Verification items for the finished model (mm, model axes). A direction names the side the tool comes from. Round coordinates to 2 decimals unless told otherwise and drop trailing zeros. Order: outer loops, then holes, each group sorted by start corner. A loop starts at its lowest first (then second) coordinate and runs counter-clockwise, first axis right, second up. Notation, with made-up numbers: (7.25, 74) -> (66.25, 74) arc R25 cw to (66.25, 97) -> close; hole circle Ø11 at (22.5, -11). An arc over 180 degrees is marked (long way). Answer in a Markdown table with one row per item. Add a question column.
```python
from build123d import *

# Parameters (mm, degrees)
EXTRUDE_1_DEPTH     = 15
CUT_EXTRUDE_1_DEPTH = 14
SKETCH_7_W          = 48
SKETCH_7_H          = 6
CUT_EXTRUDE_2_DEPTH = 1
SKETCH_8_W          = 14
SKETCH_8_H          = 4
CUT_EXTRUDE_3_DEPTH = 1


with BuildPart() as part:
    # 草图3 → 凸台-拉伸1 (new body)
    with BuildSketch(Plane.XY):
        Polygon((-26, 21.5), (24, 21.5), (24, 13.5), (6.5, 13.5), (6.5, 8), (17.5, 8), (17.5, -1), (12.5, -1), (12.5, -17.5), (-12.5, -17.5), (-12.5, -1), (-17.5, -1), (-17.5, 8), (-11.75, 8), (-11.75, 13.5), (-26, 13.5), align=None)
    extrude(amount=EXTRUDE_1_DEPTH)

    # 草图4 → 切除-拉伸1 (cut)
    with BuildSketch(Plane.XY.offset(15)):
        Polygon((23, 20.5), (-25, 20.5), (-25, 14.5), (-10.75, 14.5), (-10.75, 7), (-16.5, 7), (-16.5, 0), (-11.5, 0), (-11.5, -16.5), (11.5, -16.5), (11.5, 0), (16.5, 0), (16.5, 7), (5.5, 7), (5.5, 14.5), (23, 14.5), align=None)
    extrude(amount=-CUT_EXTRUDE_1_DEPTH, mode=Mode.SUBTRACT)

    # 草图7 → 切除-拉伸2 (cut)
    with BuildSketch(Plane.XY.offset(1)):
        with Locations((-1, 17.5)):
            Rectangle(SKETCH_7_W, SKETCH_7_H)
    extrude(amount=-CUT_EXTRUDE_2_DEPTH, mode=Mode.SUBTRACT)

    # 草图8 → 切除-拉伸3 (cut)
    with BuildSketch(Plane.ZY.offset(12.5)):
        with Locations((8, -12.5)):
            Rectangle(SKETCH_8_W, SKETCH_8_H)
    extrude(amount=-CUT_EXTRUDE_3_DEPTH, mode=Mode.SUBTRACT)


solid = part.part
```
1) Cross-section at B-B, the plane y = 16.5. Record the boundary of the cut face in (x, z).
2) Thickness scan on L1, parallel to Y at x = -14.5, z = 10; L2, parallel to Y at x = 15.5, z = 0.75; L3, parallel to Y at x = 7, z = 1.5. Record the ranges inside material, lowest first. Write a range as [from, to].
3) Cross-section at D-D, the plane y = 12.5. Record the boundary of the cut face in (x, z).
4) Cross-section at A-A, the plane x = 2.5. Record the boundary of the cut face in (y, z), and give its area (3 significant figures).
5) Cross-section at C-C, the plane y = -6. Record the boundary of the cut face in (x, z), and give its area (3 significant figures).
6) Depth check by flat-ended pin: P1, Ø1.6, axis at y = 11, z = 8, coming from the -X side; P2, Ø4, axis at y = -9.5, z = 9.5, coming from the -X side; P3, Ø1, axis at y = 6, z = 13, coming from the -X side. Enter the tip coordinate at first touch or a pass-through.
7) Draft check along X on faces 1 (the face through (24, 18, 7)), 2 (the face through (-26, 17, 7)), 3 (the face through (14, 0, 8)), 4 (the face through (9, 14.5, 8)). Enter one of: +X half, -X half, draft (parallel to the pull), parting line (faces both ways), or undercut.
8) Tool access check on faces 5 (the face through (-11.75, 11, 7)), 6 (the face through (12, 8, 7)), 7 (the face through (-15, -1, 7)), 8 (the face through (-12, -10.5, 8)), 9 (the face through (5.5, 11, 8)). Record the directions out of +Z, -Z, +X, -X, +Y, -Y that give a thin tool (end or side, any length) a straight path to the whole face; none if there is none.
Results below:
| question | item | result |
|---|---|---|
| 1 | outline | (-26, 0) -> (-25, 0) -> (-25, 15) -> (-26, 15) -> close; (23, 0) -> (24, 0) -> (24, 15) -> (23, 15) -> close |
| 2 | L1 | [-1, 0], [7, 8], [13.5, 14.5], [20.5, 21.5] |
| 2 | L2 | [-1, 8], [13.5, 14.5], [20.5, 21.5] |
| 2 | L3 | [-17.5, -16.5], [7, 8], [13.5, 14.5], [20.5, 21.5] |
| 3 | outline | (-11.75, 0) -> (6.5, 0) -> (6.5, 15) -> (5.5, 15) -> (5.5, 1) -> (-10.75, 1) -> (-10.75, 15) -> (-11.75, 15) -> close |
| 4 | outline | (-17.5, 0) -> (14.5, 0) -> (14.5, 1) -> (-16.5, 1) -> (-16.5, 15) -> (-17.5, 15) -> close; (20.5, 0) -> (21.5, 0) -> (21.5, 15) -> (20.5, 15) -> close |
| 4 | area | 61.0 mm² |
| 5 | outline | (-12.5, 0) -> (12.5, 0) -> (12.5, 15) -> (11.5, 15) -> (11.5, 1) -> (-11.5, 1) -> (-11.5, 15) -> (-12.5, 15) -> close |
| 5 | area | 53.0 mm² |
| 6 | P1 | x = -11.75 |
| 6 | P2 | x = -12.5 |
| 6 | P3 | x = -17.5 |
| 7 | face 1 | +X half |
| 7 | face 2 | -X half |
| 7 | face 3 | undercut |
| 7 | face 4 | undercut |
| 8 | face 5 | +Z, -Z, -X |
| 8 | face 6 | +Z, -Z, +X |
| 8 | face 7 | +Z, -Z, -X, -Y |
| 8 | face 8 | +Z, -X |
| 8 | face 9 | +Z |
